CAD build for the part. Positions are in the model's coordinates, mm. A direction names the side the tool comes from. Coordinates: 2 decimals unless noted, no trailing zeros. Order: outer loops, then holes, each group sorted by start corner. A loop starts at its lowest first (then second) coordinate and runs counter-clockwise, first axis right, second up. Notation, with made-up numbers: (85.5, 38.5) - (89.5, 38.5) arc R24 ccw to (89.5, 74.5) - close; hole circle Ø9 at (64.5, 65). An arc over 180 degrees is marked (long way). Write each question's results on one line, items separated by ' | '. Start each with the question number.
Q1. Wall check: probe 1 along X at (y, z) = (-7.5, 6.35); probe 2 along Y at (x, z) = (65, 12); probe 3 along Z at (x, y) = (80, -5). Give the ranges that are in metal, low to high.
Q2. Band-saw the part on A-A, the plane x = 38.5. Write the cut outline in (y, z), then the cut area to 3 significant figures.
Q3. Pull direction Z, two halves, no side cores. Call faces 1 (the flat face through (43, -137, 0)), 2 (the flat face through (43, -226.6, 6)), 3 (the cylindrical face through (14.152, -218.551, 5.372)): released by +Z, released by -Z, zero draft, split by the parting line, or undercut.
Q4. Pin check, flat tips, straight feed: P1, Ø8, axis at x = 15, y = -146, coming from the -Z side; P2, Ø4, axis at x = 48.26, z = 6.35, coming from the -Y side; P3, Ø3, axis at x = 48.26, z = 6.35, coming from the +Y side; P4, Ø3, axis at x = 80.01, z = 6.35, coming from the -Y side. Stop position of each tip, or through.
Q5. Which spindle directions (+Z, -Z, +X, -X, +Y, -Y) get a long thin tool onto all of the face, cutting with end or side? Do faces 4 (the flat face through (43, -188.909, 6)), 5 (the flat face through (86.36, -112, 6)), 6 (the cylindrical face through (18.868, -8.049, 5.372)), 7 (the cylindrical face through (50.29, -218.55, 4.8)). Say none if no direction does.
```python
from build123d import *

# Parameters (mm, degrees)
F0_W     = 86.36
F0_H     = 12.7
F1_DEPTH = 226.6
F3_D     = 8.8
F6_D     = 5.1054
F6_DEPTH = 15.875
F6_TIP   = 1.5338169022
F8_D     = 5.1054
F8_DEPTH = 15.875
F8_TIP   = 1.5338169022
F9_DEPTH = 25.4


# Not quite as in the source:
# - a feature names something its author has since deleted; it is built from what else it names


with BuildPart() as f1:
    # F0 (on Front) → F1 (new body)
    with BuildSketch(Plane.XZ):
        with Locations((43.18, 6.35)):
            Rectangle(F0_W, F0_H)
    extrude(amount=F1_DEPTH)

    # F3 (through all)
    with Locations(Plane.XY.offset(12.7)):
        with Locations((19.05, -113.29949), (65.405, -113.29949), (65.405, -33.28949), (19.05, -193.30949), (65.405, -193.30949), (19.05, -33.28949)):
            Hole(F3_D / 2)

    # F6
    with Locations(Plane.XZ.offset(226.6)):
        with Locations((16.51, 6.35), (48.26, 6.35), (80.01, 6.35)):
            Hole(F6_D / 2, depth=F6_DEPTH)
            with Locations((0, 0, -(F6_DEPTH + F6_TIP / 2))):  # 118° drill point
                Cone(0, F6_D / 2, F6_TIP, mode=Mode.SUBTRACT)

    # F8
    with Locations(Plane(origin=(0, 0, 0), x_dir=(-1, 0, 0), z_dir=(0, 1, 0))):
        with Locations((-80.01, 6.35), (-48.26, 6.35), (-16.51, 6.35)):
            Hole(F8_D / 2, depth=F8_DEPTH)
            with Locations((0, 0, -(F8_DEPTH + F8_TIP / 2))):  # 118° drill point
                Cone(0, F8_D / 2, F8_TIP, mode=Mode.SUBTRACT)

    # F4 (on face) → F9 (cut)
    with BuildSketch(Plane.XY.offset(12.7)):
        with BuildLine():
            ThreePointArc((23.45, -193.30949), (22.1612698372, -196.4207598372), (19.05, -197.70949))
            Line((19.05, -197.70949), (65.405, -197.70949))
            ThreePointArc((65.405, -197.70949), (61.005, -193.30949), (65.405, -188.90949))
            Line((65.405, -188.90949), (19.05, -188.90949))
            ThreePointArc((19.05, -188.90949), (22.1612698372, -190.1982201628), (23.45, -193.30949))
        make_face()
        with BuildLine():
            ThreePointArc((65.405, -117.69949), (61.005, -113.29949), (65.405, -108.89949))
            Line((65.405, -108.89949), (19.05, -108.89949))
            ThreePointArc((19.05, -108.89949), (22.1612698372, -110.1882201628), (23.45, -113.29949))
            ThreePointArc((23.45, -113.29949), (22.1612698372, -116.4107598372), (19.05, -117.69949))
            Line((19.05, -117.69949), (65.405, -117.69949))
        make_face()
        with BuildLine():
            ThreePointArc((65.405, -37.68949), (61.005, -33.28949), (65.405, -28.88949))
            Line((65.405, -28.88949), (19.05, -28.88949))
            ThreePointArc((19.05, -28.88949), (22.1612698372, -30.1782201628), (23.45, -33.28949))
            ThreePointArc((23.45, -33.28949), (22.1612698372, -36.4007598372), (19.05, -37.68949))
            Line((19.05, -37.68949), (65.405, -37.68949))
        make_face()
    extrude(amount=-F9_DEPTH, mode=Mode.SUBTRACT)


solid = f1.part
```
Results below:
1) probe 1: x = 0 to 13.96, 19.06 to 45.71, 50.81 to 77.46, 82.56 to 86.36 | probe 2: y = -226.6 to -197.71, -188.91 to -117.7, -108.9 to -37.69, -28.89 to 0 | probe 3: z = 0 to 3.8, 8.9 to 12.7
2) outline: (-226.6, 0) - (-197.71, 0) - (-197.71, 12.7) - (-226.6, 12.7) - close; (-188.91, 0) - (-117.7, 0) - (-117.7, 12.7) - (-188.91, 12.7) - close; (-108.9, 0) - (-37.69, 0) - (-37.69, 12.7) - (-108.9, 12.7) - close; (-28.89, 0) - (0, 0) - (0, 12.7) - (-28.89, 12.7) - close | area: 2,540 mm²
3) face 1: released by -Z | face 2: zero draft | face 3: undercut
4) P1: stops at z = 0 | P2: stops at y = -210.39 | P3: stops at y = -16.51 | P4: stops at y = -210.09
5) face 4: +Z, -Z | face 5: +Z, -Z, +X, +Y, -Y | face 6: +Y | face 7: -Y
